Model file for the job. Use its own axes, mm. Give positions to 0.01 mm unless a question says otherwise; leave off trailing zeros. Loops run counter-clockwise (first coordinate to the right, second up) from the corner with the lowest first, then second, coordinate; pieces in that order, holes last. Notation, with made-up numbers: (-5, 34.5) - (20, 34.5) arc R38 ccw to (20, 73.5) - close; hole circle Ø11 at (80, -33.75). An arc over 180 degrees is marked (long way). Answer as CSV lines item,"result". Start each with the question number.
Item 1: Drill centre lines: L1, parallel to Z at x = -187.5, y = 1.3; L2, parallel to X at y = 2, z = 362.5; L3, parallel to X at y = 0.8, z = 115 (3 decimals). Where is each one in solid material? Low to high. Write a range as from..to.
Item 2: Saw through at A-A on x = -129. Give the cut face in (y, z) (3 decimals).
Item 3: Saw through at C-C on z = 153. Give the cut face in (x, y) (3 decimals), plus the area to 3 significant figures.
Item 4: Saw through at B-B on y = 1.9. State how many separate pieces and enclosed holes the cut face has, plus the area to 3 significant figures.
Item 5: Pin check, flat tips, straight feed: pin 1 (6.5 mm diameter, centred on x = -187.5, z = 115, fed in from +Y) (3 decimals); pin 2 (5 mm diameter, centred on x = -187.5, z = 235, fed in from -Y). Stop position of each tip, or through.
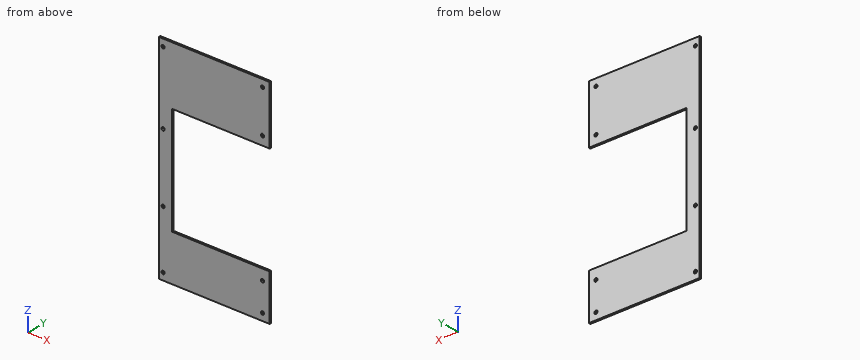
from build123d import *

# Parameters (mm, degrees)
SKETCH1_W           = 200
SKETCH1_H           = 100
SKETCH1_R           = 2.8
SKETCH1_W_2         = 175
SKETCH1_H_2         = 75
BOSS_EXTRUDE1_DEPTH = 3.175
SKETCH2_W           = 171.825
SKETCH2_H           = 6.35
BOSS_EXTRUDE2_DEPTH = 3.175
SKETCH3_W           = 5
SKETCH3_H           = 375
CUT_EXTRUDE1_DEPTH  = 426.011859393


with BuildPart() as part:
    # Sketch1 → Boss-Extrude1 (new body)
    # profile 1 of 3: a face of its own
    with BuildSketch(Plane(origin=(0, 0, 0), x_dir=(-1, 0, 0), z_dir=(0, 1, 0))):
        with Locations((100, 325)):
            Rectangle(SKETCH1_W, SKETCH1_H)
        with Locations(Location((187.5, 362.5, 0), (0, 0, 90))):
            Circle(SKETCH1_R, mode=Mode.SUBTRACT)
        with Locations(Location((12.5, 287.5, 0), (0, 0, 90))):
            Circle(SKETCH1_R, mode=Mode.SUBTRACT)
        with Locations(Location((12.5, 362.5, 0), (0, 0, 90))):
            Circle(SKETCH1_R, mode=Mode.SUBTRACT)
    # profile 2 of 3: a face of its own
    with BuildSketch(Plane(origin=(0, 0, 0), x_dir=(-1, 0, 0), z_dir=(0, 1, 0))):
        Polygon((200, 275), (175, 275), (175, 75), (175, 0), (200, 0), align=None)
        with Locations(Location((187.5, 12.5, 0), (0, 0, 90))):
            Circle(SKETCH1_R, mode=Mode.SUBTRACT)
        with Locations(Location((187.5, 115, 0), (0, 0, 90))):
            Circle(SKETCH1_R, mode=Mode.SUBTRACT)
        with Locations(Location((187.5, 235, 0), (0, 0, 90))):
            Circle(SKETCH1_R, mode=Mode.SUBTRACT)
    # profile 3 of 3: a face of its own
    with BuildSketch(Plane(origin=(0, 0, 0), x_dir=(-1, 0, 0), z_dir=(0, 1, 0))):
        with Locations((87.5, 37.5)):
            Rectangle(SKETCH1_W_2, SKETCH1_H_2)
        with Locations(Location((12.5, 12.5, 0), (0, 0, 90))):
            Circle(SKETCH1_R, mode=Mode.SUBTRACT)
        with Locations(Location((12.5, 62.5, 0), (0, 0, 90))):
            Circle(SKETCH1_R, mode=Mode.SUBTRACT)
    extrude(amount=BOSS_EXTRUDE1_DEPTH)

    # Sketch2 → Boss-Extrude2 (add, through all)
    with BuildSketch(Plane(origin=(0, 3.175, 0), x_dir=(-1, 0, 0), z_dir=(0, 1, 0))):
        Polygon((175, 275), (0, 275), (0, 271.825), (171.825, 271.825), (175, 271.825), align=None)
        Polygon((175, 75), (175, 271.825), (171.825, 271.825), (171.825, 81.35), (171.825, 75), align=None)
        with Locations((85.9125, 78.175)):
            Rectangle(SKETCH2_W, SKETCH2_H)
    extrude(amount=-BOSS_EXTRUDE2_DEPTH)

    # Sketch3 → Cut-Extrude1 (cut, through all)
    with BuildSketch(Plane(origin=(0, 3.175, 0), x_dir=(-1, 0, 0), z_dir=(0, 1, 0))):
        with Locations((197.5, 187.5)):
            Rectangle(SKETCH3_W, SKETCH3_H)
    extrude(amount=-CUT_EXTRUDE1_DEPTH, mode=Mode.SUBTRACT)


solid = part.part
Responses:
1,L1,"0..9.7, 15.3..112.2, 117.8..232.2, 237.8..359.7, 365.3..375"
1,L2,"-195..-190.3, -184.7..-15.3, -9.7..0"
1,L3,"-195..-190.3, -184.7..-171.825"
2,outline,"(0, 0) - (3.175, 0) - (3.175, 81.35) - (0, 81.35) - close; (0, 271.825) - (3.175, 271.825) - (3.175, 375) - (0, 375) - close"
3,outline,"(-195, 0) - (-171.825, 0) - (-171.825, 3.175) - (-195, 3.175) - close"
3,area,"73.6 mm2"
4,separate pieces,"1"
4,enclosed holes,"8"
4,area,"40,200 mm2"
5,pin 1,"y = 3.175"
5,pin 2,"through"
